Input: dimensioned drawing with shaded views. Units: mm. Origin: part minimum x, y, z. A direction names the side the tool comes from. Round coordinates to 2 decimals unless told otherwise and drop trailing zeros. Loops run counter-clockwise (first coordinate to the right, second up) from the corner with the lowest first, then second, coordinate; pieces in that order, holes last.
Item 1: Section query B-B on x = 7. Return loops of the section in (y, z), then the cut area to 3 significant figures.
Item 2: Section query A-A on y = 7. Return loops of the section in (x, z).
Item 3: Section query C-C on z = 0.75. Return loops of the section in (x, y).
Item 4: Pull-direction query (X, two-part tool) for the marked faces 3, 4 and 5; classes: released by +X, released by -X, zero draft, split by the parting line, or undercut.
Item 5: Ray query, L1, parallel to Y at x = 9, z = 3.4; L2, parallel to Z at x = 1.25, y = 6.5; L3, parallel to X at y = 6, z = 3.55. Return the intervals inside material, ascending.
Item 6: Section query D-D on x = 14.75. Return loops of the section in (y, z), then the cut area to 3 significant figures.
Item 7: Access query for the marked faces 1 and 2. Directions: +Z, -Z, +X, -X, +Y, -Y. A direction counts if a zero-diameter tool reaches every point of the face in a straight line with its end or side. Return the directions, or none.
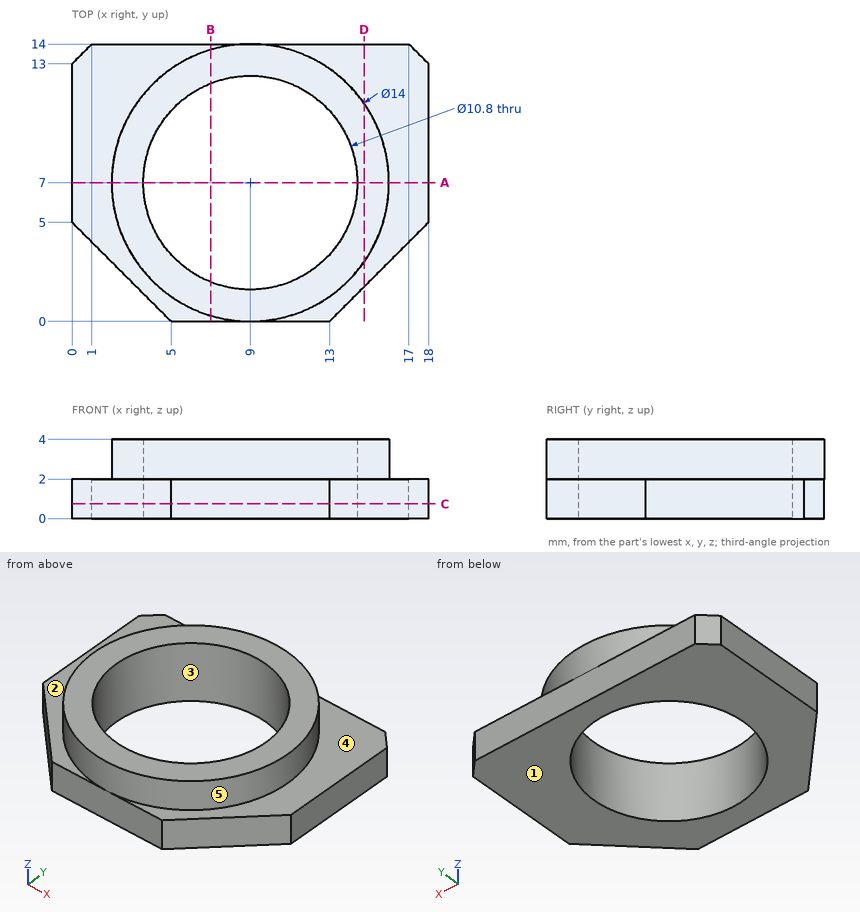
Data:
1. outline: (0, 0) - (1.98, 0) - (1.98, 4) - (0.29, 4) - (0.29, 2) - (0, 2) - close; (12.02, 0) - (14, 0) - (14, 2) - (13.71, 2) - (13.71, 4) - (12.02, 4) - close
1. area: 14.7 mm2
2. outline: (0, 0) - (3.6, 0) - (3.6, 4) - (2, 4) - (2, 2) - (0, 2) - close; (14.4, 0) - (18, 0) - (18, 2) - (16, 2) - (16, 4) - (14.4, 4) - close
3. outline: (0, 5) - (5, 0) - (13, 0) - (18, 5) - (18, 13) - (17, 14) - (1, 14) - (0, 13) - close; hole circle Ø10.8 at (9, 7)
4. face 3: undercut
4. face 4: zero draft
4. face 5: split by the parting line
5. L1: y = 0 to 1.6, 12.4 to 14
5. L2: z = 0 to 2
5. L3: x = 2.07 to 3.69, 14.31 to 15.93
6. outline: (1.75, 0) - (14, 0) - (14, 2) - (10.99, 2) - (10.99, 4) - (3.01, 4) - (3.01, 2) - (1.75, 2) - close
6. area: 40.5 mm2
7. face 1: -Z, +X, -X, +Y, -Y
7. face 2: +Z, -X
